Source: CAD feature listing. Evaluate the final solid. Frame: model axes, mm. Round coordinates to 2 decimals unless told otherwise and drop trailing zeros. Loops run counter-clockwise (first coordinate to the right, second up) from the corner with the lowest first, then second, coordinate; pieces in that order, holes last.
(1) Material intervals for probe 1 along X at (y, z) = (-1.4, 121); probe 2 along Z at (x, y) = (115.5, -1.1); probe 3 along Z at (x, y) = (30, -0.8), sorted ascending.
(2) First-contact query: pin 1 Ø0.9 at (y, z) = (-1.5, 106) entering from -X; pin 2 Ø1.5 at (x, y) = (168.5, -1) entering from -Z; pin 3 Ø1.5 at (y, z) = (-1, 127) entering from +X. Flat tips, straight axial feed; report the tip coordinate or a pass-through.
(3) Section B-B, the plane y = -1.6. Return the cut outline in (x, z), plus the area to 3 significant figures.
(4) Section C-C, the plane x = 95. Return the cut outline in (y, z).
(5) Section D-D, the plane z = 90.5. Return the cut outline in (x, y).
(6) Section A-A, the plane x = 122.5. Return the cut outline in (y, z).
```python
from build123d import *

# Parameters (mm, degrees)
F0_W     = 30
F0_H     = 3
F0_W_2   = 3
F0_H_2   = 30
F1_DEPTH = 3
F2_W     = 48
F2_H     = 38
F2_W_2   = 3
F2_H_2   = 30
F3_DEPTH = 25


with BuildPart() as f1:
    # F0 (on Front) → F1 (new body)
    with BuildSketch(Plane.XZ):
        Polygon((0, 67), (0, 0), (68.5, 0), (98.5, 0), (167, 0), (167, 88.5), (167, 118.5), (167, 143.5), (106, 143.5), (106, 67), align=None)
        with Locations((83.5, -1.5)):
            Rectangle(F0_W, F0_H)
        with Locations((168.5, 103.5)):
            Rectangle(F0_W_2, F0_H_2)
    extrude(amount=F1_DEPTH)

    # F2 (on face) → F3 (cut)
    with BuildSketch(Plane.XZ.offset(3)):
        with Locations((136.5, 116.5)):
            Rectangle(F2_W, F2_H)
        with Locations((107.5, 103.5)):
            Rectangle(F2_W_2, F2_H_2)
    extrude(amount=-F3_DEPTH, mode=Mode.SUBTRACT)


solid = f1.part
```
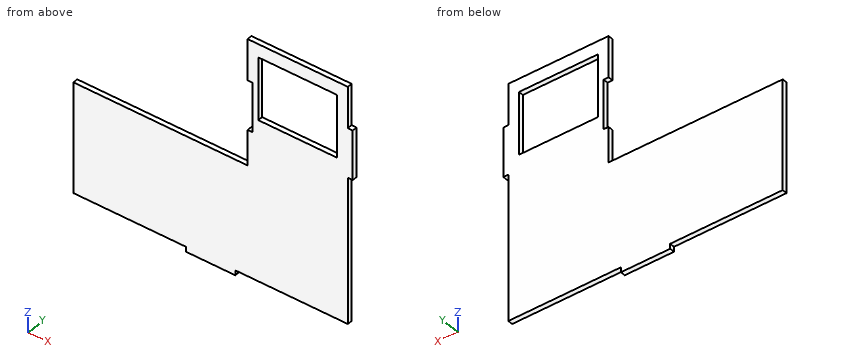
Output values:
1. probe 1: x = 106 to 112.5, 160.5 to 167
1. probe 2: z = 0 to 97.5, 135.5 to 143.5
1. probe 3: z = 0 to 67
2. pin 1: stops at x = 109
2. pin 2: stops at z = 88.5
2. pin 3: stops at x = 167
3. outline: (0, 0) - (68.5, 0) - (68.5, -3) - (98.5, -3) - (98.5, 0) - (167, 0) - (167, 88.5) - (170, 88.5) - (170, 118.5) - (167, 118.5) - (167, 143.5) - (106, 143.5) - (106, 118.5) - (109, 118.5) - (109, 88.5) - (106, 88.5) - (106, 67) - (0, 67) - close; hole (112.5, 97.5) - (160.5, 97.5) - (160.5, 135.5) - (112.5, 135.5) - close
3. area: 14,100 mm2
4. outline: (-3, -3) - (0, -3) - (0, 67) - (-3, 67) - close
5. outline: (109, -3) - (170, -3) - (170, 0) - (109, 0) - close
6. outline: (-3, 0) - (0, 0) - (0, 97.5) - (-3, 97.5) - close; (-3, 135.5) - (0, 135.5) - (0, 143.5) - (-3, 143.5) - close
